from build123d import *

# Parameters (mm, degrees)
BOSS_EXTRUDE1_DEPTH = 3.175
SKETCH3_W           = 3.3782
SKETCH3_H           = 9.116578424
CUT_EXTRUDE2_DEPTH  = 4.175


with BuildPart() as part:
    # Sketch2 → Boss-Extrude1 (new body)
    with BuildSketch(Plane.XY):
        with BuildLine():
            Line((0, -94.469447024), (0, -81.769447024))
            ThreePointArc((0, -81.769447024), (45.478698707, -101.330055673), (93.98, -111.257453101))
            ThreePointArc((93.98, -111.257453101), (246.131127604, -118.387559898), (398.184073829, -109.403930433))
            ThreePointArc((398.184073829, -109.403930433), (494.24795915, -93.166461028), (588.593285498, -68.858337449))
            Line((588.593285498, -68.858337449), (590.864339182, -81.353629169))
            ThreePointArc((590.864339182, -81.353629169), (496.73811025, -108.348158667), (400.203586987, -124.765753327))
            ThreePointArc((400.203586987, -124.765753327), (247.132802315, -132.883361709), (93.98, -126.497453101))
            ThreePointArc((93.98, -126.497453101), (45.293757409, -115.460746442), (0, -94.469447024))
        make_face()
    extrude(amount=BOSS_EXTRUDE1_DEPTH)

    # Sketch3 → Cut-Extrude2 (cut, through all)
    with BuildSketch(Plane.XY.offset(3.175)):
        Polygon((0, -81.823651503), (0, -88.181271503), (3.302, -88.181271503), (3.302, -81.823651503), (3.302, -80.849253243), (0, -80.849253243), align=None)
        with Locations((93.98, -112.972963904)):
            Rectangle(SKETCH3_W, SKETCH3_H)
        Polygon((183.426070396, 128.229599916), (183.158711139, 134.615096468), (186.330931782, 134.747916609), (186.598291039, 128.362420058), align=None)
        Polygon((193.849633474, -123.151114373), (197.224876239, -123.009793743), (196.926348208, -115.879875231), (193.551105443, -116.021195861), align=None)
        Polygon((397.375099539, -116.299780406), (400.723885221, -115.854954941), (399.211318768, -104.467880056), (395.862533086, -104.912705522), align=None)
        Polygon((295.823280702, -123.008827736), (299.189034058, -122.719104443), (298.52739573, -115.032765525), (295.161642374, -115.322488818), align=None)
        Polygon((586.515324681, -75.768921214), (589.838721446, -75.162893837), (588.533193274, -68.003500927), (585.209796509, -68.609528304), align=None)
        Polygon((496.875793957, -99.221011682), (500.199190722, -98.614984306), (498.73195058, -90.568778264), (495.408553815, -91.174805641), align=None)
    extrude(amount=-CUT_EXTRUDE2_DEPTH, mode=Mode.SUBTRACT)


solid = part.part
Input: part model. Units: mm. Frame: model coordinates. A direction names the side the tool comes from. Round coordinates to 2 decimals unless told otherwise and drop trailing zeros. Write each loop counter-clockwise with the first axis right and the second up, starting at its lowest first coordinate (ties: lowest second). Pieces come first, ordered by that corner, then holes.
1) Contact query for flat-ended pins moving along their axis: P1, Ø1.6, axis at x = 93.5, z = 2, coming from the +Y side; P2, Ø1, axis at x = 452, z = 0.5, coming from the -Y side; P3, Ø10, axis at x = 93.5, y = -115.5, coming from the -Z side. Output: stop coordinate, or through.
2) Draft query along X for faces 3 (the cylindrical face through (46, -115.7, 1.6)), 4 (the flat face through (297, -127, 0)), 5 (the cylindrical face through (45.838, -101.443, 1.565)). Return one class per face: pulls with the +X half, pulls with the -X half, needs draft (parallel to the pull), parting line crosses it, or undercut.
3) Reachability of faces 1 (the cylindrical face through (541.84, -81.97, 1.57)), 2 (the flat face through (297, -127, 3.175)) from +Z, -Z, +X, -X, +Y, -Y: full face, straight path, thin tool, end or side. Return the list, or none.
4) Ray query, L1, parallel to Y at x = 386, z = 1.25; L2, parallel to Y at x = 240, z = 0.55. Return the intervals inside material, ascending.
5) Cut plane B-B (x = 120.5). Return the cut outline in (y, z) (3 decimals), then the cut area to 3 significant figures.
6) Cut plane C-C (x = 188). Return the cut outline in (y, z) (3 decimals), then the cut area to 3 significant figures.
Geometry says:
1. P1: stops at y = -117.53
1. P2: stops at y = -117.41
1. P3: stops at z = 0
2. face 3: pulls with the -X half
2. face 4: needs draft
2. face 5: undercut
3. face 1: +Z, -Z, +Y
3. face 2: +Z, +X, -X, +Y, -Y
4. L1: y = -126.13 to -110.72
4. L2: y = -132.91 to -118.41
5. outline: (-128.645, 0) - (-113.664, 0) - (-113.664, 3.175) - (-128.645, 3.175) - close
5. area: 47.6 mm2
6. outline: (-132.138, 0) - (-117.568, 0) - (-117.568, 3.175) - (-132.138, 3.175) - close
6. area: 46.3 mm2
